Geometry: final body of the model. Coordinates: model frame, mm. Give positions to 0.01 mm unless a question says otherwise; leave off trailing zeros. Loops run counter-clockwise (first coordinate to the right, second up) from the corner with the lowest first, then second, coordinate; pieces in that order, holes last. Notation, with made-up numbers: (3.25, 5.5) -> (7.25, 5.5) arc R9 ccw to (7.25, 12.5) -> close; hole circle Ø4 at (-40, 39). An arc over 180 degrees is marked (long way). One line per item, written item: value. Start each with the question number.
from build123d import *

# Parameters (mm, degrees)
SZKIC1_R                    = 4.5
SZKIC1_R_2                  = 0.5
DODANIE_WYCI_GNI_CIE1_DEPTH = 3
SZKIC2_R                    = 0.5
WYTNIJ_WYCI_GNI_CIE1_DEPTH  = 1


with BuildPart() as part:
    # Szkic1 → Dodanie-wyciągnięcie1 (new body)
    with BuildSketch(Plane.XY):
        Circle(SZKIC1_R)
        Circle(SZKIC1_R_2, mode=Mode.SUBTRACT)
    extrude(amount=DODANIE_WYCI_GNI_CIE1_DEPTH)

    # Szkic2 → Wytnij-wyciągnięcie1 (cut)
    with BuildSketch(Plane.XY.offset(3)):
        with Locations((0, 3.625)):
            Circle(SZKIC2_R)
        with Locations((1.572828554, 3.266012146)):
            Circle(SZKIC2_R)
        with Locations((2.834139124, 2.260150532)):
            Circle(SZKIC2_R)
        with Locations((3.534113682, 0.806638386)):
            Circle(SZKIC2_R)
        with Locations((3.534113682, -0.806638386)):
            Circle(SZKIC2_R)
        with Locations((2.834139124, -2.260150532)):
            Circle(SZKIC2_R)
        with Locations((1.572828554, -3.266012146)):
            Circle(SZKIC2_R)
        with Locations((0, -3.625)):
            Circle(SZKIC2_R)
        with Locations((-1.572828554, -3.266012146)):
            Circle(SZKIC2_R)
        with Locations((-2.834139124, -2.260150532)):
            Circle(SZKIC2_R)
        with Locations((-3.534113682, -0.806638386)):
            Circle(SZKIC2_R)
        with Locations((-3.534113682, 0.806638386)):
            Circle(SZKIC2_R)
        with Locations((-2.834139124, 2.260150532)):
            Circle(SZKIC2_R)
        with Locations((-1.572828554, 3.266012146)):
            Circle(SZKIC2_R)
    extrude(amount=-WYTNIJ_WYCI_GNI_CIE1_DEPTH, mode=Mode.SUBTRACT)


solid = part.part
Item 1: Section A-A, the plane x = 0. Output: boundary loops of the cut face in (y, z) (3 decimals), then the cut area to 3 significant figures.
Item 2: Pin query (flat end, axial travel): pin 1 (0.5 mm diameter, centred on x = 0, y = 3.5, fed in from +Z). Return the tip coordinate at first contact, or that it passes through.
Item 3: Section B-B, the plane y = 0. Output: boundary loops of the cut face in (x, z).
Item 4: Ray query, line 1 along Y through (x, z) = (0, 2.25) (3 decimals); line 2 along Y through (x, z) = (0, 1.15); line 3 along X through (y, z) = (2, 2.1). Return the intervals inside material, ascending. Write a range as [from, to].
Item 5: Section C-C, the plane z = 0.9. Output: boundary loops of the cut face in (x, y), then the cut area to 3 significant figures.
Item 6: Mould query, pull axis Y, two halves, no side actions, for faces 1 (the face through (0, -1, 3)), 2 (the face through (3.166, 1.145, 2.507)). Classes: pulls with the +Y half, pulls with the -Y half, needs draft (parallel to the pull), parting line crosses it, or undercut.
Item 7: Section D-D, the plane y = 4. Output: boundary loops of the cut face in (x, z).
Geometry check:
1. outline: (-4.5, 0) -> (-0.5, 0) -> (-0.5, 3) -> (-3.125, 3) -> (-3.125, 2) -> (-4.125, 2) -> (-4.125, 3) -> (-4.5, 3) -> close; (0.5, 0) -> (4.5, 0) -> (4.5, 3) -> (4.125, 3) -> (4.125, 2) -> (3.125, 2) -> (3.125, 3) -> (0.5, 3) -> close
1. area: 22.0 mm2
2. pin 1: stops at z = 2
3. outline: (-4.5, 0) -> (-0.5, 0) -> (-0.5, 3) -> (-4.5, 3) -> close; (0.5, 0) -> (4.5, 0) -> (4.5, 3) -> (0.5, 3) -> close
4. line 1: y = [-4.5, -4.125], [-3.125, -0.5], [0.5, 3.125], [4.125, 4.5]
4. line 2: y = [-4.5, -0.5], [0.5, 4.5]
4. line 3: x = [-4.03, -3.26], [-2.41, 2.41], [3.26, 4.03]
5. outline: circle Ø9 at (0, 0); hole circle Ø1 at (0, 0)
5. area: 62.8 mm2
6. face 1: needs draft
6. face 2: undercut
7. outline: (-2.06, 0) -> (2.06, 0) -> (2.06, 3) -> (0.33, 3) -> (0.33, 2) -> (-0.33, 2) -> (-0.33, 3) -> (-2.06, 3) -> close
